Part model, mm, in its own coordinate system. Face numbers are marked on the shaded views. A direction names the side the tool comes from. Give positions to 0.01 mm unless a question says otherwise; leave off trailing zeros. Order: outer loops, then holes, each group sorted by start corner. A loop starts at its lowest first (then second) coordinate and runs counter-clockwise, first axis right, second up. Notation, with made-up numbers: M 66.25,42.5 L 89.25,42.5 A23 ccw 89.25,67.5 Z; hole C 15,-7 d5. An arc over 180 degrees is marked long. Answer as a JSON object with one key per item and string values.
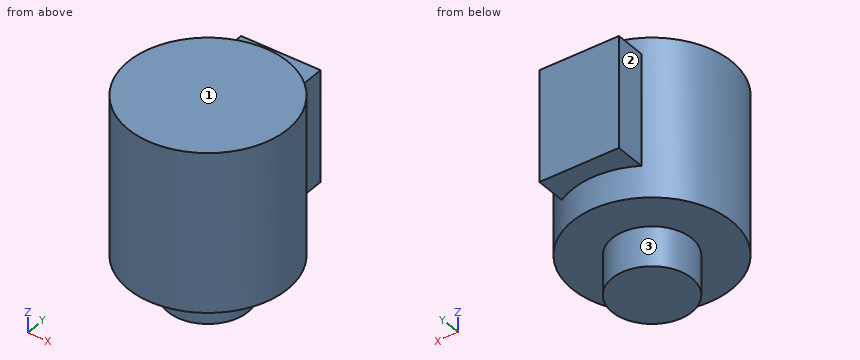
from build123d import *

# Parameters (mm, degrees)
SKETCH_1_R      = 10
EXTRUDE_1_DEPTH = 10
SKETCH_2_R      = 20
EXTRUDE_2_DEPTH = 40
SKETCH_3_W      = 20
SKETCH_3_H      = 28
EXTRUDE_3_DEPTH = 25


with BuildPart() as part:
    # 草图1 → 凸台-拉伸1 (new body)
    with BuildSketch(Plane.XY):
        Circle(SKETCH_1_R)
    extrude(amount=EXTRUDE_1_DEPTH)

    # 草图2 → 凸台-拉伸2 (add)
    with BuildSketch(Plane.XY.offset(10)):
        Circle(SKETCH_2_R)
    extrude(amount=EXTRUDE_2_DEPTH)

    # 草图3 → 凸台-拉伸3 (add)
    with BuildSketch(Plane(origin=(0, 0, 0), x_dir=(1, 0, 0), z_dir=(0, 1, 0))):
        with Locations((0, -32)):
            Rectangle(SKETCH_3_W, SKETCH_3_H)
    extrude(amount=EXTRUDE_3_DEPTH)


solid = part.part
1. Cut at B-B on y = 0. Give the cut face in (x, z).
Worked answers:
{"outline": "M -20,10 L -10,10 L -10,0 L 10,0 L 10,10 L 20,10 L 20,50 L -20,50 Z"}
2. Cut at A-A on x = 0. Give the cut face in (y, z), plus the area to 3 significant figures.
Worked answers:
{"outline": "M -20,10 L -10,10 L -10,0 L 10,0 L 10,10 L 20,10 L 20,18 L 25,18 L 25,46 L 20,46 L 20,50 L -20,50 Z", "area": "1,940 mm^2"}
3. Probe line 1 along X through (y, z) = (20, 37); line 2 along Z through (x, y) = (14, 5.5); line 3 along Y through (x, z) = (-5, 44.5). List the from-to ranges inside material, lowest first.
Worked answers:
{"line 1": "x = -10 to 10", "line 2": "z = 10 to 50", "line 3": "y = -19.36 to 25"}
4. Which spindle directions (+Z, -Z, +X, -X, +Y, -Y) get a long thin tool onto all of the face, cutting with end or side? Do the marked faces 1, 2 and 3. Say none if no direction does.
Worked answers:
{"face 1": "+Z, +X, -X, +Y, -Y", "face 2": "+Z, -Z, -X, +Y", "face 3": "-Z"}
5. Cut at C-C on z = 17. Give the cut face in (x, y), plus the area to 3 significant figures.
Worked answers:
{"outline": "C 0,0 d40", "area": "1,260 mm^2"}
6. Pin check, flat tips, straight feed: P1, Ø3, axis at x = 3, z = 38, coming from the -Y side; P2, Ø5, axis at y = 14, z = 18, coming from the +X side; P3, Ø10, axis at x = 0, z = 32.5, coming from the -Y side. Stop position of each tip, or through.
Worked answers:
{"P1": "stops at y = -19.94", "P2": "stops at x = 16.36", "P3": "stops at y = -20"}
7. Cut at D-D on x = -7.5. Give the cut face in (y, z), plus the area to 3 significant figures.
Worked answers:
{"outline": "M -18.54,10 L -6.61,10 L -6.61,0 L 6.61,0 L 6.61,10 L 18.54,10 L 18.54,18 L 25,18 L 25,46 L 18.54,46 L 18.54,50 L -18.54,50 Z", "area": "1,800 mm^2"}
